Model file for the job. Use its own axes, mm. Face numbers are marked on the shaded views. Round coordinates to 2 decimals unless told otherwise and drop trailing zeros. Use one line per item in the form item = value.
from build123d import *

# Parameters (mm, degrees)
CUT_EXTRUDE4_DEPTH  = 1.905
SKETCH15_R          = 2.286
BOSS_EXTRUDE3_DEPTH = 2.54
SKETCH17_R          = 0.889
CUT_EXTRUDE5_DEPTH  = 3.81
CUT_EXTRUDE6_DEPTH  = 0.9525
CUT_EXTRUDE9_DEPTH  = 205.915011065


with BuildPart() as part:
    # Sketch2 → Loft3 section 0
    with BuildSketch(Plane(origin=(0, 0, 0), x_dir=(1, 0, 0), z_dir=(0, 1, 0))):
        with BuildLine():
            Line((153.170003889, 0), (183.992068321, 11.558274162))
            Line((183.992068321, 11.558274162), (183.992068321, 78.611725838))
            Line((183.992068321, 78.611725838), (153.170003889, 90.17))
            Line((153.170003889, 90.17), (142.590068321, 90.17))
            Line((142.590068321, 90.17), (142.590068321, 0))
            Line((142.590068321, 0), (153.170003889, 0))
        make_face()
    # Sketch3 → Loft3 section 1
    with BuildSketch(Plane(origin=(0, 3.81, 0), x_dir=(1, 0, 0), z_dir=(0, 1, 0))):
        with BuildLine():
            Line((142.590068321, 3.81), (142.590068321, 86.36))
            Line((142.590068321, 86.36), (152.479119132, 86.36))
            Line((152.479119132, 86.36), (180.182068321, 75.971394054))
            Line((180.182068321, 75.971394054), (180.182068321, 14.198605946))
            Line((180.182068321, 14.198605946), (152.479119132, 3.81))
            Line((152.479119132, 3.81), (142.590068321, 3.81))
        make_face()
    loft()

    # Sketch14 → Cut-Extrude4 (cut)
    with BuildSketch(Plane(origin=(0, 3.81, 0), x_dir=(1, 0, 0), z_dir=(0, 1, 0))):
        Polygon((178.277068321, 74.651228162), (152.133676754, 84.455), (144.495068321, 84.455), (144.495068321, 5.715), (152.133676754, 5.715), (178.277068321, 15.518771838), align=None)
    extrude(amount=-CUT_EXTRUDE4_DEPTH, mode=Mode.SUBTRACT)

    # Sketch15 → Boss-Extrude3 (add)
    with BuildSketch(Plane(origin=(0, 1.905, 0), x_dir=(1, 0, 0), z_dir=(0, 1, 0))):
        with Locations(Location((173.959068321, 61.9252, 0), (0, 0, 270))):
            Circle(SKETCH15_R)
        with Locations(Location((147.162068321, 46.3042, 0), (0, 0, 270))):
            Circle(SKETCH15_R)
        with Locations(Location((156.991868321, 28.2702, 0), (0, 0, 270))):
            Circle(SKETCH15_R)
    extrude(amount=BOSS_EXTRUDE3_DEPTH)

    # Sketch17 → Cut-Extrude5 (cut)
    with BuildSketch(Plane(origin=(0, 4.445, 0), x_dir=(1, 0, 0), z_dir=(0, 1, 0))):
        with Locations(Location((156.991868321, 28.2702, 0), (0, 0, 270))):
            Circle(SKETCH17_R)
        with Locations(Location((147.162068321, 46.3042, 0), (0, 0, 270))):
            Circle(SKETCH17_R)
        with Locations(Location((173.959068321, 61.9252, 0), (0, 0, 270))):
            Circle(SKETCH17_R)
    extrude(amount=-CUT_EXTRUDE5_DEPTH, mode=Mode.SUBTRACT)

    # Sketch18 → Cut-Extrude6 (cut)
    with BuildSketch(Plane(origin=(0, 3.81, 0), x_dir=(1, 0, 0), z_dir=(0, 1, 0))):
        Polygon((179.229568321, 14.858688892), (179.229568321, 75.311311108), (152.306397943, 85.4075), (143.542568321, 85.4075), (143.542568321, 4.7625), (152.306397943, 4.7625), align=None)
        Polygon((178.277068321, 15.518771838), (178.277068321, 74.651228162), (152.133676754, 84.455), (144.495068321, 84.455), (144.495068321, 5.715), (152.133676754, 5.715), align=None, mode=Mode.SUBTRACT)
    extrude(amount=-CUT_EXTRUDE6_DEPTH, mode=Mode.SUBTRACT)

    # Sketch22 → Cut-Extrude9 (cut, through all)
    with BuildSketch(Plane(origin=(0, 1.905, 0), x_dir=(1, 0, 0), z_dir=(0, 1, 0))):
        with BuildLine():
            ThreePointArc((170.657068321, 21.209), (169.579437586, 20.762630735), (169.133068321, 19.685))
            Line((169.133068321, 19.685), (170.657068321, 19.685))
            Line((170.657068321, 19.685), (170.657068321, 21.209))
        make_face()
        with BuildLine():
            Line((170.657068321, 19.685), (169.133068321, 19.685))
            ThreePointArc((169.133068321, 19.685), (170.657068321, 18.161), (172.181068321, 19.685))
            ThreePointArc((172.181068321, 19.685), (171.734699055, 20.762630735), (170.657068321, 21.209))
            Line((170.657068321, 21.209), (170.657068321, 19.685))
        make_face()
        with BuildLine():
            ThreePointArc((151.607068321, 21.209), (150.529437586, 18.607369265), (153.131068321, 19.685))
            Line((153.131068321, 19.685), (151.607068321, 19.685))
            Line((151.607068321, 19.685), (151.607068321, 21.209))
        make_face()
        with BuildLine():
            Line((151.607068321, 19.685), (153.131068321, 19.685))
            ThreePointArc((153.131068321, 19.685), (152.684699055, 20.762630735), (151.607068321, 21.209))
            Line((151.607068321, 21.209), (151.607068321, 19.685))
        make_face()
        with BuildLine():
            ThreePointArc((169.133068321, 70.485), (169.579437586, 69.407369265), (170.657068321, 68.961))
            Line((170.657068321, 68.961), (170.657068321, 70.485))
            Line((170.657068321, 70.485), (169.133068321, 70.485))
        make_face()
        with BuildLine():
            Line((170.657068321, 70.485), (170.657068321, 68.961))
            ThreePointArc((170.657068321, 68.961), (171.734699055, 69.407369265), (172.181068321, 70.485))
            ThreePointArc((172.181068321, 70.485), (170.657068321, 72.009), (169.133068321, 70.485))
            Line((169.133068321, 70.485), (170.657068321, 70.485))
        make_face()
        with BuildLine():
            ThreePointArc((153.131068321, 70.485), (150.529437586, 71.562630735), (151.607068321, 68.961))
            Line((151.607068321, 68.961), (151.607068321, 70.485))
            Line((151.607068321, 70.485), (153.131068321, 70.485))
        make_face()
        with BuildLine():
            Line((151.607068321, 70.485), (151.607068321, 68.961))
            ThreePointArc((151.607068321, 68.961), (152.684699055, 69.407369265), (153.131068321, 70.485))
            Line((153.131068321, 70.485), (151.607068321, 70.485))
        make_face()
    extrude(amount=-CUT_EXTRUDE9_DEPTH, mode=Mode.SUBTRACT)


solid = part.part
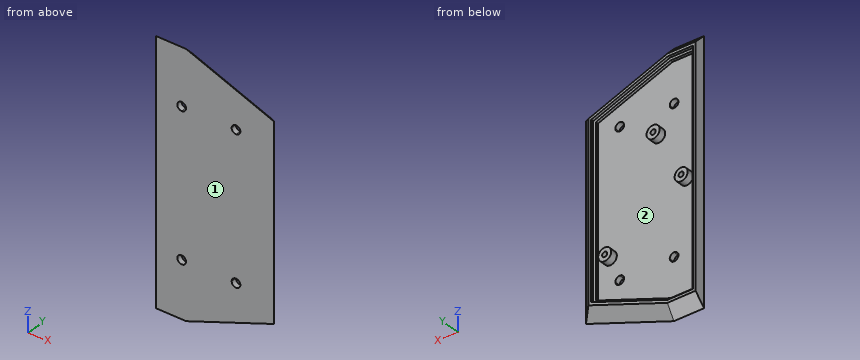
1. Pull direction X, two halves, no side cores. Call the marked faces 1 and 2: +X half, -X half, draft (parallel to the pull), parting line (faces both ways), or undercut.
Geometry check:
face_1 = draft
face_2 = undercut
2. Wall check: probe 1 along Y at (x, z) = (149.5, -6) (3 decimals); probe 2 along X at (y, z) = (3.4, -48); probe 3 along X at (y, z) = (2.95, -66.5). Give the ranges that are in metal, low to high.
Geometry check:
probe_1 = 0 to 1.905
probe_2 = 142.59 to 143.54, 145.63 to 148.7, 179.23 to 180.59
probe_3 = 142.59 to 143.54, 179.23 to 181.04
3. Flat gauge pins, fed straight in: pin 1 (10 mm diameter, centred on x = 158.5, z = -43, fed in from +Y) (3 decimals); pin 2 (2 mm diameter, centred on y = 2, z = -32.5, fed in from +X); pin 3 (12 mm diameter, centred on x = 150, z = -34.5, fed in from +Y). Where does each tip first touch, or does it go through?
Geometry check:
pin_1 = 1.905
pin_2 = 182.99
pin_3 = 2.86
